Drawing for the job (mm, zero at the part's lowest x, y, z). A direction names the side the tool comes from. Round coordinates to 2 decimals unless told otherwise and drop trailing zeros. Order: outer loops, then holes, each group sorted by start corner. A loop starts at its lowest first (then second) coordinate and runs counter-clockwise, first axis right, second up. Notation, with made-up numbers: (-23, -34.5) - (36, -34.5) arc R8 cw to (36, -21.5) - close; hole circle Ø11 at (-7.5, 4.25). An arc over 180 degrees is marked (long way). Answer as a JSON object with one key per item and string values.
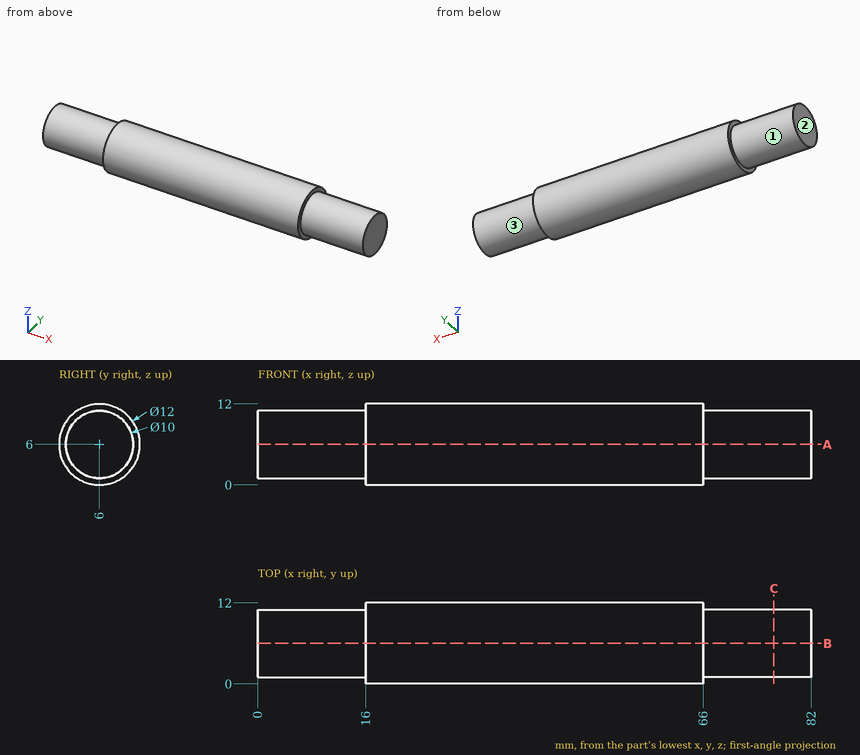
Item 1: Cut at A-A (z = 6). Write the cut outline in (x, y), plus the area to 3 significant figures.
Taken from the geometry:
{"outline": "(0, 1) - (16, 1) - (16, 0) - (66, 0) - (66, 1) - (82, 1) - (82, 11) - (66, 11) - (66, 12) - (16, 12) - (16, 11) - (0, 11) - close", "area": "920 mm2"}
Item 2: Probe L1, parallel to X at y = 1.25, z = 9; L2, parallel to Y at x = 27, z = 5.25; L3, parallel to Y at x = 54.5, z = 0.75. List the from-to ranges inside material, lowest first. Write a range as from..to.
Taken from the geometry:
{"L1": "16..66", "L2": "0.05..11.95", "L3": "3.1..8.9"}
Item 3: Tool access for the marked faces 1, 2 and 3: list every direction of +Z, -Z, +X, -X, +Y, -Y with a clear straight run to the whole face (end or side of a thin tool).
Taken from the geometry:
{"face 1": "-X", "face 2": "+Z, -Z, -X, +Y, -Y", "face 3": "+X"}
Item 4: Drop flat-ended pins along their axis: P1, Ø5, axis at x = 59.5, z = 1.5, coming from the +Y side; P2, Ø1, axis at x = 32, y = 9.5, coming from the -Z side; P3, Ø3, axis at x = 53.5, y = 9.5, coming from the +Z side. Give the stop position or say it passes through.
Taken from the geometry:
{"P1": "y = 11.66", "P2": "z = 0.8", "P3": "z = 11.66"}
Item 5: Cut at C-C (x = 76.5). Write the cut outline in (y, z).
Taken from the geometry:
{"outline": "circle Ø10 at (6, 6)"}
